Autodesk Inventor part; units mm, degrees
ref_plane "YZ Plane" through (0, 0, 0) normal (1, 0, 0) x (0, 1, 0)
ref_plane "XZ Plane" through (0, 0, 0) normal (0, 1, 0) x (-1, 0, 0)
ref_plane "XY Plane" through (0, 0, 0) normal (0, 0, 1) x (1, 0, 0)
sketch "Sketch1" plane through (0, 0, 0) normal (0, 0, 1) x (1, 0, 0)
  line L0 (-13.202, 13.202) -> (12.198, 13.202)
  line L1 (12.198, 13.202) -> (12.198, -12.198)
  line L2 (12.198, -12.198) -> (-13.202, -12.198)
  line L3 (-13.202, -12.198) -> (-13.202, 13.202)
  point P0 (0, 0)
  dimension "d0" = 25.4
  dimension "d1" = 25.4
extrude "Extrusion1" add sketch "Sketch1" along normal blind 101.6
sketch "Sketch6" plane through (12.198, 13.202, 101.6) normal (1, 0, 0) x (0, 0, -1)
  line L0 (101.6, 0) -> (101.6, -25.4)
  line L1 (101.6, -25.4) -> (0, -25.4)
  line L2 (101.6, 0) -> (101.6, -25.4)
  line L3 (101.6, 0) -> (0, 0)
  line L4 (0, -25.4) -> (0, 0)
  line L5 (0, -25.4) -> (0, 0)
  point P0 (101.6, -13.202)
  point P1 (88.9, -6.35)
  point P2 (88.9, -19.05)
  point P3 (101.6, -19.05)
  point P4 (101.6, -6.35)
  point P5 (12.7, -6.35)
  point P6 (12.7, -19.05)
  point P7 (0, -19.05)
  point P8 (0, -6.35)
  dimension "d51" = 12.7
  dimension "d52" = 6.35
  dimension "d53" = 12.7
  dimension "d54" = 6.35
  dimension "d55" = 12.7
  dimension "d56" = 6.35
  dimension "d57" = 12.7
  dimension "d58" = 6.35
hole "Hole5" at (12.198, 6.852, 12.7) at (12.198, -5.848, 12.7) at (12.198, 6.852, 88.9) at (12.198, -5.848, 88.9) direction (-1, 0, 0) diameter 4.318 end through all counterbore diameter 7.62 counterbore depth 4.318
sketch "Sketch9" plane through (-13.202, 13.202, 0) normal (0, 1, 0) x (1, 0, 0)
  line L0 (0, 0) -> (0, -101.6)
  line L1 (0, 0) -> (25.4, 0)
  line L2 (25.4, -101.6) -> (0, -101.6)
  point P0 (13.202, 0)
  point P1 (12.7, -25.4)
  point P2 (12.7, -76.2)
  dimension "d101" = 12.7
  dimension "d102" = 12.7
  dimension "d103" = 25.4
  dimension "d104" = 25.4
hole "Hole6" at (-0.502, 13.202, 25.4) at (-0.502, 13.202, 76.2) direction (0, -1, 0) diameter 4.4958 end through all
sketch "Sketch10" plane through (12.198, -12.198, 0) normal (1, 0, 0) x (0, 0, -1)
  line L0 (-101.6, 0) -> (-101.6, 25.4)
  line L1 (0, 25.4) -> (0, 0)
  line L2 (0, 0) -> (-101.6, 0)
  point P0 (0, 12.198)
  point P1 (-63.5, 5.08)
  point P2 (-38.1, 5.08)
  dimension "d112" = 38.1
  dimension "d113" = 38.1
  dimension "d114" = 5.08
  dimension "d115" = 5.08
hole "Hole7" at (12.198, -7.118, 63.5) at (12.198, -7.118, 38.1) direction (-1, 0, 0) diameter 6.7564 end through all
properties part number "BackEndSlider"
Input: part model. Units: mm. Frame: model coordinates. A direction names the side the tool comes from. Give positions to 0.01 mm unless a question says otherwise; leave off trailing zeros. Order: outer loops, then holes, each group sorted by start corner. A loop starts at its lowest first (then second) coordinate and runs counter-clockwise, first axis right, second up. Notation, with made-up numbers: M 4.5,17 L 57.5,17 A28 ccw 57.5,52 Z; hole C 67,47.5 d8. An arc over 180 degrees is marked long. Return JSON: item names as keys, results as strings.
Item 1: Cut plane D-D (x = -11.5). Return loops of the section in (y, z), then the cut area to 3 significant figures.
Solutions:
{"outline": "M -12.2,0 L 13.2,0 L 13.2,101.6 L -12.2,101.6 Z; hole C -7.12,38.1 d6.76; hole C -7.12,63.5 d6.76; hole C -5.85,12.7 d4.32; hole C -5.85,88.9 d4.32; hole C 6.85,12.7 d4.32; hole C 6.85,88.9 d4.32", "area": "2,450 mm^2"}
Item 2: Access query for faces 1 (the flat face through (7.88, -4, 87)), 2 (the cylindrical face through (-2.809, 6.757, 91.057)). Directions: +Z, -Z, +X, -X, +Y, -Y. A direction counts if a zero-diameter tool reaches every point of the face in a straight line with its end or side. Return the directions, or none.
Solutions:
{"face 1": "+X", "face 2": "+X, -X"}
Item 3: Cut plane C-C (z = 63.5). Return loops of the section in (x, y), then the cut area to 3 significant figures.
Solutions:
{"outline": "M -13.2,-12.2 L 12.2,-12.2 L 12.2,-10.5 L -13.2,-10.5 Z; M -13.2,-3.74 L 12.2,-3.74 L 12.2,13.2 L -13.2,13.2 Z", "area": "474 mm^2"}
Item 4: Cut plane A-A (z = 25.4). Return loops of the section in (x, y).
Solutions:
{"outline": "M -13.2,-12.2 L -2.75,-12.2 L -2.75,13.2 L -13.2,13.2 Z; M 1.75,-12.2 L 12.2,-12.2 L 12.2,13.2 L 1.75,13.2 Z"}
Item 5: Pull-direction query (Y, two-part tool) for faces 3 (the flat face through (12.198, 1, 50)), 4 (the cylindrical face through (-2.81, 8.96, 13.17)), 5 (the flat face through (0, -12.198, 50)); classes: +Y half, -Y half, draft (parallel to the pull), parting line (faces both ways), or undercut.
Solutions:
{"face 3": "draft", "face 4": "undercut", "face 5": "-Y half"}
Item 6: Cut plane B-B (z = 88.9). Return loops of the section in (x, y), then the cut area to 3 significant figures.
Solutions:
{"outline": "M -13.2,-12.2 L 12.2,-12.2 L 12.2,-9.66 L 7.88,-9.66 L 7.88,-8.01 L -13.2,-8.01 Z; M -13.2,-3.69 L 7.88,-3.69 L 7.88,-2.04 L 12.2,-2.04 L 12.2,3.04 L 7.88,3.04 L 7.88,4.69 L -13.2,4.69 Z; M -13.2,9.01 L 7.88,9.01 L 7.88,10.66 L 12.2,10.66 L 12.2,13.2 L -13.2,13.2 Z", "area": "397 mm^2"}
Item 7: Ray query, probe 1 along Y at (x, z) = (9.1, 12.7); probe 2 along Z at (x, y) = (-7.5, 6); probe 3 along Z at (x, y) = (-9.75, -7). Return the intervals inside material, ascending.
Solutions:
{"probe 1": "-12.2 to -9.66, -2.04 to 3.04, 10.66 to 13.2", "probe 2": "0 to 10.72, 14.68 to 86.92, 90.88 to 101.6", "probe 3": "0 to 10.87, 14.53 to 34.72, 41.48 to 60.12, 66.88 to 87.07, 90.73 to 101.6"}
Item 8: First-contact query: P1, Ø6, axis at y = -5.848, z = 88.9, coming from the +X side. Flat tip, straight axial feed; report the tip coordinate or a pass-through.
Solutions:
{"P1": "x = 7.88"}
